Design review of the part built by this model. Coordinates are the model's own, in mm. Face numbers are marked on the shaded views. A direction names the side the tool comes from. Coordinates: 2 decimals unless noted, no trailing zeros. Write each loop counter-clockwise with the first axis right and the second up, starting at its lowest first coordinate (ties: lowest second). Pieces come first, ordered by that corner, then holes. Notation, with made-up numbers: (44, -17) -> (70, -17) arc R15 ccw to (70, -7) -> close; hole circle Ø5 at (79, 18). An arc over 180 degrees is marked (long way). One line per question, with ' | ' between items. Start each with the question number.
Q1. For the marked faces 5, 6 and 7, list the 3-axis set-ups (+Z, -Z, +X, -X, +Y, -Y) from which the entire face can be reached by the end or side of a thin tool; tool diameter is ignored.
Q2. Add section A-A on x = 5.25. State the section outline as (y, z) points, and give its area (3 significant figures).
Q3. For P1, Ø1.6, axis at x = 26.52, y = -6.78, coming from the +Z side; P2, Ø1.5, axis at y = -5, z = 3.5, coming from the -X side, all flat-tipped, find the tip position at first contact; note any pin that passes through.
Q4. Draft analysis for pull direction X (two halves, no side actions). For the marked faces 1, 2, 3 and 4, state which applies: pulls with the +X half, pulls with the -X half, needs draft (parallel to the pull), parting line crosses it, or undercut.
Q5. Wall thickness on probe 1 along Z at (x, y) = (9.5, -4); probe 2 along X at (y, z) = (-3, 1.5); probe 3 along X at (y, z) = (-4, 5.5): over which ranges is each line inside the solid? List them lowest first.
from build123d import *

# Parameters (mm, degrees)
SKETCH2_R           = 0.500109693
BOSS_EXTRUDE1_DEPTH = 5
BOSS_EXTRUDE2_DEPTH = 1


with BuildPart() as part:
    # Sketch2 → Boss-Extrude1 (new body)
    with BuildSketch(Plane(origin=(0, 0, 0), x_dir=(1, 0, 0), z_dir=(0, 0, -1))):
        with BuildLine():
            Line((29.97295835, 6.642737104), (28.862437793, 5.215722686))
            Line((28.862437793, 5.215722686), (29.97295835, 3.953817374))
            add(Edge.make_bspline(
                [(5.565346412, 3.953817374), (17.919076804, -3.939717318), (29.97295835, 3.953817374)],
                knots=[0, 0, 0, 1, 1, 1], degree=2))
            Line((5.565346412, 3.953817374), (0, 0.570103483))
            Line((0, 0.570103483), (2.65645961, 5.215722686))
            Line((2.65645961, 5.215722686), (0, 9.556126627))
            Line((0, 9.556126627), (5.565346412, 6.285726684))
            add(Edge.make_bspline(
                [(5.565346412, 6.285726684), (12.037313538, 11.217277608), (22.14175538, 12.07873787), (29.97295835, 6.642737104)],
                knots=[0, 0, 0, 0, 1, 1, 1, 1], degree=3))
        make_face()
        with Locations(Location((26.5225963, 6.780666166, 0), (0, 0, 180))):
            Circle(SKETCH2_R, mode=Mode.SUBTRACT)
    extrude(amount=-BOSS_EXTRUDE1_DEPTH)

    # Sketch4 → Boss-Extrude2 (add)
    with BuildSketch(Plane(origin=(0, 0, 5), x_dir=(-1, 0, 0), z_dir=(0, 0, 1))):
        with BuildLine():
            Line((-13.908305334, 1.34956402), (-13.908305334, 9.133973525))
            Line((-13.908305334, 9.133973525), (-16.004621445, 9.133973525))
            Line((-16.004621445, 9.133973525), (-16.004621445, 5.241768773))
            add(Edge.make_bspline(
                [(-16.004621445, 5.241768773), (-16.954182776, 5.785448359), (-18.2214925, 8.172395217), (-18.647004572, 8.368785404)],
                knots=[0, 0, 0, 0, 1, 1, 1, 1], degree=3))
            add(Edge.make_bspline(
                [(-18.647004572, 8.368785404), (-19.182278095, 8.856654309), (-19.866173762, 9.102220728), (-20.698347409, 9.084883777)],
                knots=[0, 0, 0, 0, 1, 1, 1, 1], degree=3))
            add(Edge.make_bspline(
                [(-20.698347409, 9.084883777), (-22.350260741, 9.040072434), (-23.33079469, 7.762774595), (-23.476488694, 5.241768773)],
                knots=[0, 0, 0, 0, 1, 1, 1, 1], degree=3))
            add(Edge.make_bspline(
                [(-20.404496328, 1.575368175), (-22.334339213, 1.71536757), (-23.381711079, 2.669128019), (-23.476488694, 5.241768773)],
                knots=[0, 0, 0, 0, 1, 1, 1, 1], degree=3))
            Line((-20.404496328, 1.575368175), (-20.223319436, 4.140832963))
            add(Edge.make_bspline(
                [(-21.56956029, 5.431442564), (-21.582844794, 4.484850448), (-20.84335959, 4.096124714), (-20.223319436, 4.140832963)],
                knots=[0, 0, 0, 0, 1, 1, 1, 1], degree=3))
            add(Edge.make_bspline(
                [(-20.623882844, 6.487488573), (-21.093503681, 6.435159023), (-21.557848723, 6.102593618), (-21.56956029, 5.431442564)],
                knots=[0, 0, 0, 0, 1, 1, 1, 1], degree=3))
            add(Edge.make_bspline(
                [(-19.082560895, 5.639341249), (-19.40985103, 6.125934593), (-20.210193184, 6.544584723), (-20.623882844, 6.487488573)],
                knots=[0, 0, 0, 0, 1, 1, 1, 1], degree=3))
            add(Edge.make_bspline(
                [(-13.908305334, 1.34956402), (-16.125553437, 1.670916535), (-17.437876782, 3.20471995), (-19.082560895, 5.639341249)],
                knots=[0, 0, 0, 0, 1, 1, 1, 1], degree=3))
        make_face()
    extrude(amount=BOSS_EXTRUDE2_DEPTH)


solid = part.part
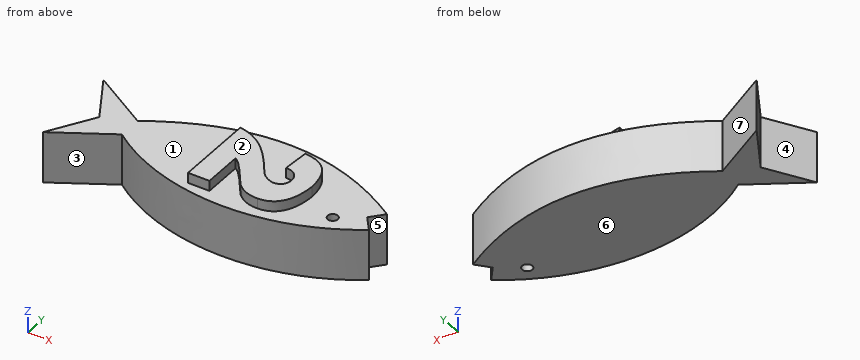
Output values:
1) face 5: +Z, -Z, +X | face 6: -Z, +X, -X, +Y, -Y | face 7: +Z, -Z, +Y
2) outline: (-6.47, 0) -> (-3.76, 0) -> (-3.76, 5) -> (-6.47, 5) -> close | area: 13.5 mm2
3) P1: stops at z = 5 | P2: stops at x = 2.1
4) face 1: undercut | face 2: needs draft | face 3: undercut | face 4: pulls with the -X half
5) probe 1: z = 0 to 5 | probe 2: x = 1.39 to 4, 7.16 to 28.41 | probe 3: x = 13.91 to 17.9, 20.23 to 23.33
